from build123d import *

# Parameters (mm, degrees)
F0_R     = 19.812
F1_DEPTH = 6.35
F2_R     = 3.175
F3_DEPTH = 25.4
F4_W     = 34.29
F4_H     = 26.162
F5_DEPTH = 2.54


with BuildPart() as f1:
    # F0 (on Top) → F1 (new body)
    with BuildSketch(Plane.XY):
        Circle(F0_R)
    extrude(amount=F1_DEPTH)

    # F2 (on face) → F3 (cut)
    with BuildSketch(Plane.XY.offset(6.35)):
        Circle(F2_R)
    extrude(amount=-F3_DEPTH, mode=Mode.SUBTRACT)

    # F4 (on face) → F5 (cut)
    with BuildSketch(Plane.XY.offset(6.35)):
        with Locations((3.81, -0.518704)):
            Rectangle(F4_W, F4_H)
    extrude(amount=-F5_DEPTH, mode=Mode.SUBTRACT)


solid = f1.part
Geometry check sheet. Reference: the model listing, model coordinates, mm. A direction names the side the tool comes from. Coordinates: 2 decimals unless noted, no trailing zeros. Write each loop counter-clockwise with the first axis right and the second up, starting at its lowest first coordinate (ties: lowest second). Pieces come first, ordered by that corner, then holes. Notation, with made-up numbers: (2.25, 81) -> (22.25, 81) arc R25 cw to (22.25, 120) -> close; hole circle Ø10 at (5.25, -39). An arc over 180 degrees is marked (long way). One line per question, with ' | ' between items.
1. Set-up check for faces 4 (the flat face through (-14, 3, 6.35)), 5 (the flat face through (0, -13.6, 5)): record each of +Z, -Z, +X, -X, +Y, -Y from which the full face is reachable in a straight line by a thin tool's end or side.
Answers:
face 4: +Z, +X, -X, +Y, -Y | face 5: +Z, +X
2. Thickness scan on probe 1 along Y at (x, z) = (0, 1.1) (3 decimals); probe 2 along Z at (x, y) = (-1, 12); probe 3 along Y at (x, z) = (-1, 2.5). Record the ranges inside material, lowest first. Write a range as from..to.
Answers:
probe 1: y = -19.812..-3.175, 3.175..19.812 | probe 2: z = 0..3.81 | probe 3: y = -19.79..-3.01, 3.01..19.79
3. Cross-section at A-A on y = 0. Record the cut outline in (x, z) (3 decimals), and give its area (3 significant figures).
Answers:
outline: (-19.812, 0) -> (-3.175, 0) -> (-3.175, 3.81) -> (-13.335, 3.81) -> (-13.335, 6.35) -> (-19.812, 6.35) -> close; (3.175, 0) -> (19.812, 0) -> (19.812, 3.81) -> (3.175, 3.81) -> close | area: 143 mm²
4. Cross-section at D-D on x = 8. Record the cut outline in (y, z) (3 decimals).
Answers:
outline: (-18.125, 0) -> (18.125, 0) -> (18.125, 6.35) -> (12.562, 6.35) -> (12.562, 3.81) -> (-13.6, 3.81) -> (-13.6, 6.35) -> (-18.125, 6.35) -> close
5. Depth check by flat-ended pin: pin 1 Ø1 at (x, y) = (3, 3) entering from -Z; pin 2 Ø10 at (x, y) = (-7.5, 5.5) entering from +Z; pin 3 Ø2 at (x, z) = (-10.5, 5) entering from +Y; pin 4 Ø0.8 at (y, z) = (-3.5, 5) entering from +X (3 decimals). Enter the tip coordinate at first touch or a pass-through.
Answers:
pin 1: stops at z = 0 | pin 2: stops at z = 3.81 | pin 3: stops at y = 17.39 | pin 4: stops at x = -13.335
6. Cross-section at B-B on x = 0. Record the cut outline in (y, z) (3 decimals).
Answers:
outline: (-19.812, 0) -> (-3.175, 0) -> (-3.175, 3.81) -> (-13.6, 3.81) -> (-13.6, 6.35) -> (-19.812, 6.35) -> close; (3.175, 0) -> (19.812, 0) -> (19.812, 6.35) -> (12.562, 6.35) -> (12.562, 3.81) -> (3.175, 3.81) -> close
7. Cross-section at C-C on z = 1.75. Record the cut outline in (x, y) (3 decimals), and give its area (3 significant figures).
Answers:
outline: circle Ø39.624 at (0, 0); hole circle Ø6.35 at (0, 0) | area: 1,200 mm²
8. Draft check along Y on faces 1 (the cylindrical face through (-19.793, 0.871, 3.131)), 2 (the flat face through (0, -4, 0)), 3 (the flat face through (3, 3, 3.81)). Enter one of: +Y half, -Y half, draft (parallel to the pull), parting line (faces both ways), or undercut.
Answers:
face 1: parting line | face 2: draft | face 3: undercut
